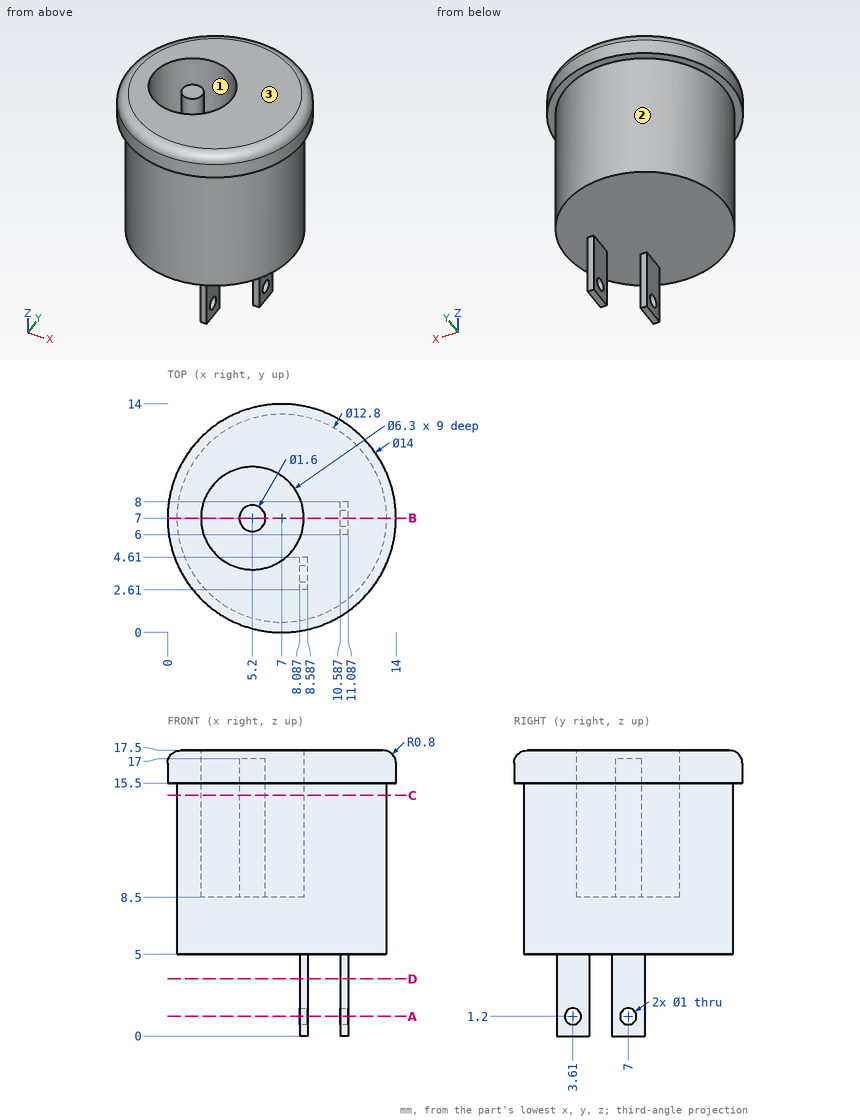
For this review, use the dimensioned drawing (mm, ordinates from the lowest corner) and the shaded views. Give positions to 0.01 mm unless a question says otherwise; leave off trailing zeros. Order: outer loops, then holes, each group sorted by start corner. A loop starts at its lowest first (then second) coordinate and runs counter-clockwise, first axis right, second up. Notation, with made-up numbers: (9.5, -7) - (66.5, -7) arc R21 ccw to (66.5, 25) - close; hole circle Ø6 at (78, 75). An arc over 180 degrees is marked (long way). Use a Markdown table: item, result. Add a question column.
(1) Add section C-C on z = 14.75. Give the boundary of the cut face in (x, y).
(2) Add section B-B on y = 7. Give the boundary of the cut face in (x, z), then the cut area to 3 significant figures.
(3) Add section A-A on z = 1.2. Give the boundary of the cut face in (x, y).
(4) Mouldability with a two-part tool opening along X and no side actions: class the marked faces 1, 2 and 3 as +X half, -X half, draft (parallel to the pull), parting line (faces both ways), or undercut.
(5) Wall thickness on probe 1 along Y at (x, z) = (10.8, 1.2); probe 2 along Y at (x, z) = (8.2, 1.2); probe 3 along Z at (x, y) = (7.75, 7.5): over which ranges is each line inside the solid? List them lowest first. Write a range as [from, to].
(6) Add section D-D on z = 3.5. Give the boundary of the cut face in (x, y).
(7) Clearance check with flat-ended pins moving along their axes: P1, Ø1, axis at y = 7, z = 1.5, coming from the +X side; P2, Ø1, axis at x = 9, z = 11.5, coming from the -Y side; P3, Ø3, axis at x = 5.5, y = 6.5, coming from the +Z side; P4, Ø6, axis at y = 7.5, z = 15.5, coming from the +X side. State where each tip first meets the part, or that it passes through.
Report:
| question | item | result |
|---|---|---|
| 1 | outline | circle Ø12.8 at (7, 7); circle Ø1.6 at (5.2, 7); hole circle Ø6.3 at (5.2, 7) |
| 2 | outline | (0, 15.5) - (0.6, 15.5) - (0.6, 5) - (10.59, 5) - (10.59, 1.7) - (11.09, 1.7) - (11.09, 5) - (13.4, 5) - (13.4, 15.5) - (14, 15.5) - (14, 16.7) arc R0.8 ccw to (13.2, 17.5) - (8.35, 17.5) - (8.35, 8.5) - (6, 8.5) - (6, 17) - (4.4, 17) - (4.4, 8.5) - (2.05, 8.5) - (2.05, 17.5) - (0.8, 17.5) arc R0.8 ccw to (0, 16.7) - close; (10.59, 0) - (11.09, 0) - (11.09, 0.7) - (10.59, 0.7) - close |
| 2 | area | 121 mm² |
| 3 | outline | (8.09, 2.61) - (8.59, 2.61) - (8.59, 3.11) - (8.09, 3.11) - close; (8.09, 4.11) - (8.59, 4.11) - (8.59, 4.61) - (8.09, 4.61) - close; (10.59, 6) - (11.09, 6) - (11.09, 6.5) - (10.59, 6.5) - close; (10.59, 7.5) - (11.09, 7.5) - (11.09, 8) - (10.59, 8) - close |
| 4 | face 1 | undercut |
| 4 | face 2 | parting line |
| 4 | face 3 | draft |
| 5 | probe 1 | y = [6, 6.5], [7.5, 8] |
| 5 | probe 2 | y = [2.61, 3.11], [4.11, 4.61] |
| 5 | probe 3 | z = [5, 8.5] |
| 6 | outline | (8.09, 2.61) - (8.59, 2.61) - (8.59, 4.61) - (8.09, 4.61) - close; (10.59, 6) - (11.09, 6) - (11.09, 8) - (10.59, 8) - close |
| 7 | P1 | stops at x = 11.09 |
| 7 | P2 | stops at y = 0.78 |
| 7 | P3 | stops at z = 17 |
| 7 | P4 | stops at x = 14 |
